Autodesk Inventor part; units mm, degrees
ref_plane "YZ Plane" through (0, 0, 0) normal (1, 0, 0) x (0, 1, 0)
ref_plane "XZ Plane" through (0, 0, 0) normal (0, 1, 0) x (-1, 0, 0)
ref_plane "XY Plane" through (0, 0, 0) normal (0, 0, 1) x (1, 0, 0)
sketch "Sketch1" plane through (0, 0, 0) normal (1, 0, 0) x (0, 1, 0)
  line L0 (0, 0) -> (120, 0)
  line L1 (120, 0) -> (120, -180)
  line L2 (120, -180) -> (0, -180)
  line L3 (0, -180) -> (0, 0)
  dimension "d0" = 120
  dimension "d1" = 180
extrude "Extrusion1" add sketch "Sketch1" along normal blind 5
sketch "Sketch2" plane through (5, 0, 0) normal (1, 0, 0) x (0, 0, -1)
  line L0 (180, 0) -> (180, 120)
  line L1 (180, 120) -> (0, 120)
  line L2 (0, 120) -> (0, 0)
  line L3 (0, 0) -> (180, 0)
  line L4 (6, 114) -> (174, 114)
  line L5 (174, 114) -> (174, 6)
  line L6 (174, 6) -> (6, 6)
  line L7 (6, 6) -> (6, 114)
  dimension "d4" = 6
extrude "Extrusion2" add sketch "Sketch2" along normal blind 45
fillet "Fillet1" radius 2 8 edges at (27.5, 114, -174) (27.5, 114, -6) (27.5, 6, -6) (27.5, 6, -174) (25, 120, -180) (25, 120, 0) (25, 0, 0) (25, 0, -180)
sketch "Sketch3" plane through (5, 0, 0) normal (1, 0, 0) x (0, 0, -1)
  circle A0 centre (15, 105) radius 1.75
  arc A1 (172, 6) -> (174, 8) centre (172, 8) ccw
  line L0 (174, 8) -> (174, 112)
  arc A2 (174, 112) -> (172, 114) centre (172, 112) ccw
  line L1 (172, 114) -> (8, 114)
  arc A3 (8, 114) -> (6, 112) centre (8, 112) ccw
  line L2 (6, 112) -> (6, 8)
  arc A4 (6, 8) -> (8, 6) centre (8, 8) ccw
  line L3 (8, 6) -> (172, 6)
  circle A5 centre (165, 105) radius 1.75
  circle A6 centre (15, 15) radius 1.75
  circle A7 centre (165, 15) radius 1.75
  line L4 (15, 105) -> (15, 114) construction
  line L5 (15, 105) -> (6, 105) construction
  line L6 (165, 15) -> (165, 6) construction
  line L7 (165, 15) -> (174, 15) construction
  point P0 (0, 0)
  dimension "d8" = 3.5
  dimension "d12" = 150
  dimension "d15" = 90
extrude "Extrusion3" cut sketch "Sketch3" against normal blind 20 contours A0 | A5 | A6 | A7
sketch "Sketch4" plane through (50, 0, 0) normal (1, 0, 0) x (0, 0, -1)
  arc A0 (178, 0) -> (180, 2) centre (178, 2) ccw
  line L0 (180, 2) -> (180, 118)
  arc A1 (180, 118) -> (178, 120) centre (178, 118) ccw
  line L1 (178, 120) -> (2, 120)
  arc A2 (2, 120) -> (0, 118) centre (2, 118) ccw
  line L2 (0, 118) -> (0, 2)
  arc A3 (0, 2) -> (2, 0) centre (2, 2) ccw
  line L3 (2, 0) -> (178, 0)
  line L4 (8, 114) -> (172, 114)
  arc A4 (174, 112) -> (172, 114) centre (172, 112) ccw
  line L5 (174, 112) -> (174, 8)
  arc A5 (172, 6) -> (174, 8) centre (172, 8) ccw
  line L6 (172, 6) -> (8, 6)
  arc A6 (6, 8) -> (8, 6) centre (8, 8) ccw
  line L7 (6, 8) -> (6, 112)
  arc A7 (8, 114) -> (6, 112) centre (8, 112) ccw
  circle A8 centre (3.5, 116.5) radius 2
  line L8 (8, 114) -> (172, 114)
  line L9 (6, 8) -> (6, 112)
  circle A9 centre (176.5, 116.5) radius 2
  circle A10 centre (176.5, 3.5) radius 2
  circle A11 centre (3.5, 3.5) radius 2
  point P0 (0, 0)
  dimension "d22" = 4
  dimension "d23" = 2.5
  dimension "d24" = 2.5
  dimension "d25" = 4
  dimension "d26" = 4
  dimension "d27" = 4
  dimension "d28" = 2.5
  dimension "d29" = 2.5
  dimension "d30" = 2.5
  dimension "d31" = 2.5
  dimension "d32" = 2.5
  dimension "d33" = 2.5
extrude "Extrusion4" cut sketch "Sketch4" against normal through all contours A8 | A9 | A10 | A11
chamfer "Chamfer1" distance 1 distance2 2 4 edges at (0, 116.5, -174.5) (0, 116.5, -1.5) (0, 3.5, -1.5) (0, 3.5, -174.5) measured on face at (0, 45.2711, -65.5165)
chamfer "Chamfer2" distance 1 distance2 2 4 edges at (50, 3.5, -174.5) (50, 3.5, -1.5) (50, 116.5, -1.5) (50, 116.5, -174.5) measured on face at (50, 3.4492, -117.3333)
chamfer "Chamfer3" distance 1 distance2 1 4 edges at (5, 105, -13.25) (5, 105, -163.25) (5, 15, -13.25) (5, 15, -163.25) measured on face at (5, 45.2711, -65.5165)
sketch "Sketch5" plane through (5, 114, -172) normal (0, -1, 0) x (1, 0, 0)
  line L0 (45, 170) -> (-5, 170)
  line L1 (45, -6) -> (45, 170)
  line L2 (-5, -6) -> (45, -6)
  line L3 (-5, -6) -> (-5, 170)
  line L4 (0, 164) -> (45, 164)
  line L5 (0, 0) -> (0, 164)
  line L6 (45, 0) -> (0, 0)
  line L7 (45, 164) -> (45, 0)
  line L8 (12, 149) -> (32, 149)
  line L9 (32, 149) -> (32, 15)
  line L10 (32, 15) -> (12, 15)
  line L11 (12, 15) -> (12, 149)
  point P0 (-5, 172)
  point P1 (22.5, 164)
  dimension "d45" = 15
  dimension "d46" = 15
  dimension "d47" = 12
  dimension "d48" = 20
extrude "Extrusion5" cut sketch "Sketch5" against normal blind 45 contours L8 L9 L10 L11
sketch "Sketch6" plane through (5, 8, -174) normal (0, 0, 1) x (1, 0, 0)
  line L0 (-5, 95.25) -> (-5, 98.75)
  line L1 (-1, 98.75) -> (-1, 95.25)
  line L2 (45, 0) -> (0, 0)
  line L3 (45, 104) -> (45, 0)
  line L4 (0, 104) -> (45, 104)
  line L5 (0, 0) -> (0, 104)
  line L6 (3, 93.25) -> (23, 93.25)
  line L7 (23, 93.25) -> (23, 38.25)
  line L8 (23, 38.25) -> (3, 38.25)
  line L9 (3, 38.25) -> (3, 93.25)
  point P0 (-5, -8)
  dimension "d51" = 3
  dimension "d52" = 55
  dimension "d53" = 2
  dimension "d54" = 20
extrude "Extrusion6" cut sketch "Sketch6" against normal through all contours L6 L7 L8 L9
sketch "Sketch7" plane through (5, 8, -6) normal (0, 0, -1) x (-1, 0, 0)
  line L0 (0, 0) -> (-45, 0)
  line L1 (0, 104) -> (0, 0)
  line L2 (-45, 104) -> (0, 104)
  line L3 (-45, 0) -> (-45, 104)
  line L4 (5, 98.75) -> (5, 95.25)
  line L5 (1, 95.25) -> (1, 98.75)
  line L6 (-8, 90.25) -> (-23, 90.25)
  line L7 (-23, 90.25) -> (-23, 45.25)
  line L8 (-23, 45.25) -> (-8, 45.25)
  line L9 (-8, 45.25) -> (-8, 90.25)
  point P0 (5, -8)
  dimension "d57" = 45
  dimension "d58" = 5
  dimension "d59" = 8
  dimension "d60" = 15
extrude "Extrusion7" cut sketch "Sketch7" against normal blind 10 contours L9 L8 L7 L6
fillet "Fillet2" radius 12 6 edges at (37, 117, -23) (37, 117, -157) (28, 98.25, -3) (28, 53.25, -3) (28, 101.25, -177) (28, 46.25, -177)
fillet "Fillet3" radius 2 6 edges at (13, 98.25, -3) (17, 117, -157) (8, 101.25, -177) (8, 46.25, -177) (13, 53.25, -3) (17, 117, -23)
equation "\"d28\" = d23"
equation "\"d29\" = d28"
equation "\"d30\" = d29"
equation "\"d31\" = d29"
equation "\"d32\" = d23"
equation "\"d33\" = d23"
properties part number "OCTOPUS_BOX"
Geometry check sheet. Reference: the model listing, model coordinates, mm. A direction names the side the tool comes from. Round coordinates to 2 decimals unless told otherwise and drop trailing zeros. Write each loop counter-clockwise with the first axis right and the second up, starting at its lowest first coordinate (ties: lowest second). Pieces come first, ordered by that corner, then holes.
Item 1: Go/stop test with flat-tipped pins: pin 1 Ø3 at (y, z) = (118, -91.5) entering from -X; pin 2 Ø12 at (y, z) = (62.5, -32.5) entering from +X. Record where each tip stops, or that it passes through.
Determined:
pin 1: stops at x = 0
pin 2: stops at x = 5
Item 2: Section check C-C (x = 34.5). Record the boundary of the cut face in (y, z).
Determined:
outline: (0, -178) arc R2 ccw to (2, -180) - (118, -180) arc R2 ccw to (120, -178) - (120, -152.33) - (114, -152.33) - (114, -172) arc R2 cw to (112, -174) - (8, -174) arc R2 cw to (6, -172) - (6, -8) arc R2 cw to (8, -6) - (112, -6) arc R2 cw to (114, -8) - (114, -27.67) - (120, -27.67) - (120, -2) arc R2 ccw to (118, 0) - (2, 0) arc R2 ccw to (0, -2) - close; hole circle Ø4 at (3.5, -176.5); hole circle Ø4 at (3.5, -3.5); hole circle Ø4 at (116.5, -176.5); hole circle Ø4 at (116.5, -3.5)
Item 3: Section check B-B (z = -104.5). Record the boundary of the cut face in (x, y), plus the area to 3 significant figures.
Determined:
outline: (0, 0) - (50, 0) - (50, 6) - (5, 6) - (5, 114) - (17, 114) - (17, 120) - (0, 120) - close; (37, 114) - (50, 114) - (50, 120) - (37, 120) - close
area: 1,020 mm2
Item 4: Section check D-D (y = 40). Record the boundary of the cut face in (x, z).
Determined:
outline: (0, -180) - (50, -180) - (50, -174) - (5, -174) - (5, -6) - (50, -6) - (50, 0) - (0, 0) - close
Item 5: Access from +Z, -Z, +X, -X, +Y, -Y to the whole of each face (thin tool, end or side, straight path). Record for faces 1 (the face through (24.39, 97.83, -177.04)), 2 (the face through (33.39, 117.04, -26.42)), 3 (the face through (0, 59, -89)), 4 (the face through (30, 59, 0)), 5 (the face through (13, 75, -3)).
Determined:
face 1: -Z
face 2: +Y
face 3: +Z, -Z, -X, +Y, -Y
face 4: +Z, +X, -X, +Y, -Y
face 5: +Z, -Z
Item 6: Section check A-A (y = 80.5). Record the boundary of the cut face in (x, z), plus the area to 3 significant figures.
Determined:
outline: (0, -180) - (8, -180) - (8, -174) - (5, -174) - (5, -6) - (13, -6) - (13, 0) - (0, 0) - close; (28, -180) - (50, -180) - (50, -174) - (28, -174) - close; (28, -6) - (50, -6) - (50, 0) - (28, 0) - close
area: 1,230 mm2
Item 7: Material ranges on line 1 along Y through (x, z) = (13.5, -176.5); line 2 along Y through (x, z) = (2, -15); line 3 along Z through (x, y) = (0.85, 105), recorded low to high.
Determined:
line 1: y = 0 to 1.5, 5.5 to 46.25, 101.25 to 114.5, 118.5 to 120
line 2: y = 0 to 13.25, 16.75 to 103.25, 106.75 to 120
line 3: z = -180 to -166.75, -163.25 to -16.75, -13.25 to 0
Item 8: Mould release check, pull along Y, two halves, no side actions. Record for faces 6 (the face through (24.39, 56.67, -2.96)), 7 (the face through (22, 117, -23)): +Y half, -Y half, draft (parallel to the pull), parting line (faces both ways), or undercut.
Determined:
face 6: undercut
face 7: draft
